Build history of the part. All positions in model axes, mm. A direction names the side the tool comes from. Give positions to 0.01 mm unless a question says otherwise; leave off trailing zeros. Loops run counter-clockwise (first coordinate to the right, second up) from the corner with the lowest first, then second, coordinate; pieces in that order, holes last. Notation, with made-up numbers: M 48,21.5 L 91,21.5 A12 cw 91,42.5 Z; hole C 76,70.5 d10. An arc over 180 degrees is marked long. Answer as a JSON object with one key per item and string values. Group by question number.
1. Mould opens along X. For faces 3 (the face through (0, 4, -1)), 4 (the face through (-14, 9, -1)), 5 (the face through (-14.9, 4.4, 44.3)) say: released by +X, released by -X, zero draft, split by the parting line, or undercut.
2. Drop flat-ended pins along their axis: pin 1 Ø3 at (y, z) = (4.5, -47.5) entering from -X; pin 2 Ø4 at (y, z) = (3, 10.5) entering from -X; pin 3 Ø3 at (y, z) = (5.5, -35) entering from -X. Give the stop position or say it passes through.
3. Slice it at B-B (z = -47.5). List the corners of the cut face in (x, y).
4. Slice it at A-A (x = -12.5). List the corners of the cut face in (y, z).
5. Drill centre lines: line 1 along Z through (x, y) = (-11, 4.5); line 2 along Z through (x, y) = (-11.5, 0.5); line 3 along X through (y, z) = (4.5, -47.5). Where is each one in solid material? Low to high. Write a range as [from, to].
6. Slice it at C-C (y = 4). List the corners of the cut face in (x, z), then the cut area to 3 significant figures.
7. 3-axis set-ups, long thin cutter, end or side, ignore diameter. For faces 1 (the face through (-30, 4, -45)), 2 (the face through (-14, 0, -1)): which of +Z, -Z, +X, -X, +Y, -Y reach the whole face in a straight line?
8. Slice it at D-D (x = -30). List the corners of the cut face in (y, z), then the cut area to 3 significant figures.
from build123d import *

# Parameters (mm, degrees)
SKETCH1_R           = 4
BOSS_EXTRUDE1_DEPTH = 9


with BuildPart() as part:
    # Sketch1 → Boss-Extrude1 (new body)
    with BuildSketch(Plane(origin=(0, 0, 0), x_dir=(1, 0, 0), z_dir=(0, 1, 0))):
        Polygon((0, 70), (0, -70), (-37, -70), (-23, -20), (-23, 0), (-23, 20), (-37, 70), align=None)
        with Locations(Location((-12.5, 47.5, 0), (0, 0, 270))):
            Circle(SKETCH1_R, mode=Mode.SUBTRACT)
        with Locations(Location((-12.5, -47.5, 0), (0, 0, 270))):
            Circle(SKETCH1_R, mode=Mode.SUBTRACT)
    extrude(amount=BOSS_EXTRUDE1_DEPTH)


solid = part.part
Established:
{
 "1": {"face 3": "released by +X", "face 4": "zero draft", "face 5": "undercut"},
 "2": {"pin 1": "stops at x = -31.12", "pin 2": "stops at x = -23", "pin 3": "stops at x = -27.62"},
 "3": {"outline": "M -30.7,0 L -16.5,0 L -16.5,9 L -30.7,9 Z; M -8.5,0 L 0,0 L 0,9 L -8.5,9 Z"},
 "4": {"outline": "M 0,-70 L 9,-70 L 9,-51.5 L 0,-51.5 Z; M 0,-43.5 L 9,-43.5 L 9,43.5 L 0,43.5 Z; M 0,51.5 L 9,51.5 L 9,70 L 0,70 Z"},
 "5": {"line 1": "z = [-70, -51.21], [-43.79, 43.79], [51.21, 70]", "line 2": "z = [-70, -51.37], [-43.63, 43.63], [51.37, 70]", "line 3": "x = [-30.7, -16.5], [-8.5, 0]"},
 "6": {"outline": "M -37,-70 L 0,-70 L 0,70 L -37,70 L -23,20 L -23,-20 Z; hole C -12.5,-47.5 d8; hole C -12.5,47.5 d8", "area": "3,820 mm^2"},
 "7": {"face 1": "-X, +Y, -Y", "face 2": "+Z, -Z, +X, -X, -Y"},
 "8": {"outline": "M 0,-70 L 9,-70 L 9,-45 L 0,-45 Z; M 0,45 L 9,45 L 9,70 L 0,70 Z", "area": "450 mm^2"}
}
